Check sheet for the modelled part. Datum: model origin and axes. Units: mm. A direction names the side the tool comes from. Round coordinates to 2 decimals unless told otherwise and drop trailing zeros. Write each loop counter-clockwise with the first axis right and the second up, starting at its lowest first coordinate (ties: lowest second). Pieces come first, ordered by that corner, then holes. Notation, with made-up numbers: (41.25, -9.75) -> (52.25, -9.75) arc R20 ccw to (52.25, 4.25) -> close; hole circle Ø5 at (37, 17.5). An arc over 180 degrees is marked (long way). One line per item, written item: value.
from build123d import *

# Parameters (mm, degrees)
BOSS_EXTRUDE1_DEPTH = 5
SKETCH2_R           = 7.075
SKETCH2_R_2         = 2
CUT_EXTRUDE1_DEPTH  = 5
FILLET1_R           = 10
FILLET2_R           = 10


with BuildPart() as part:
    # Sketch1 → Boss-Extrude1 (new body)
    with BuildSketch(Plane(origin=(0, 0, 0), x_dir=(1, 0, 0), z_dir=(0, 1, 0))):
        Polygon((-40.926174497, 16.946308725), (-88.926174497, 16.946308725), (-88.926174497, -33.053691275), (-40.926174497, -33.053691275), (-40.926174497, -8.053691275), (-30.926174497, -8.053691275), (-13.571066073, -8.053691275), (21.073825503, -8.053691275), (21.073825503, 46.946308725), (-30.926174497, 46.946308725), (-40.926174497, 46.946308725), align=None)
    extrude(amount=BOSS_EXTRUDE1_DEPTH)

    # Sketch2 → Cut-Extrude1 (cut)
    with BuildSketch(Plane(origin=(0, 5, 0), x_dir=(1, 0, 0), z_dir=(0, 1, 0))):
        with Locations(Location((-64.926174497, -9.053691275, 0), (0, 0, 270))):
            Circle(SKETCH2_R)
        with Locations(Location((-72.926174497, -1.053691275, 0), (0, 0, 270))):
            Circle(SKETCH2_R_2)
        with Locations(Location((-56.926174497, -1.053691275, 0), (0, 0, 270))):
            Circle(SKETCH2_R_2)
        with Locations(Location((-56.926174497, -17.053691275, 0), (0, 0, 270))):
            Circle(SKETCH2_R_2)
        with Locations(Location((-72.926174497, -17.053691275, 0), (0, 0, 270))):
            Circle(SKETCH2_R_2)
        with Locations(Location((-2.926174497, 23.643183553, 0), (0, 0, 270))):
            Circle(SKETCH2_R)
        with Locations(Location((5.073825503, 31.643183553, 0), (0, 0, 270))):
            Circle(SKETCH2_R_2)
        with Locations(Location((-10.926174497, 15.643183553, 0), (0, 0, 270))):
            Circle(SKETCH2_R_2)
        with Locations(Location((-10.926174497, 31.643183553, 0), (0, 0, 270))):
            Circle(SKETCH2_R_2)
        with Locations(Location((5.073825503, 15.643183553, 0), (0, 0, 270))):
            Circle(SKETCH2_R_2)
    extrude(amount=-CUT_EXTRUDE1_DEPTH, mode=Mode.SUBTRACT)

    # Fillet1
    fillet1_edges = [part.edges().sort_by_distance(p)[0] for p in [
        (-88.926174497, 2.5, -16.946308725),
    ]]
    fillet(fillet1_edges, radius=FILLET1_R)

    # Fillet2
    fillet2_edges = [part.edges().sort_by_distance(p)[0] for p in [
        (21.073825503, 2.5, -46.946308725),
        (21.073825503, 2.5, 8.053691275),
        (-40.926174497, 2.5, 8.053691275),
        (-40.926174497, 2.5, 33.053691275),
        (-88.926174497, 2.5, 33.053691275),
        (-40.926174497, 2.5, -16.946308725),
        (-40.926174497, 2.5, -46.946308725),
    ]]
    fillet(fillet2_edges, radius=FILLET2_R)


solid = part.part
Item 1: Sectioned sample at B-B (z = -22.5). Enter the section's corners in (x, y).
Result set:
outline: (-41.97, 0) -> (-9.91, 0) -> (-9.91, 5) -> (-41.97, 5) -> close; (4.06, 0) -> (21.07, 0) -> (21.07, 5) -> (4.06, 5) -> close
Item 2: Sectioned sample at D-D (x = -23.5). Enter the section's corners in (y, z).
Result set:
outline: (0, -46.95) -> (5, -46.95) -> (5, 8.05) -> (0, 8.05) -> close
Item 3: Release check for a two-part mould opening along Z. For faces 1 (the flat face through (-40.926, 2, 21)), 2 (the cylindrical face through (-71.2, 2.54, 12.32)), 3 (the cylindrical face through (-43.93, 2.54, 30.2)) record: pulls with the +Z half, pulls with the -Z half, needs draft (parallel to the pull), parting line crosses it, or undercut.
Result set:
face 1: needs draft
face 2: undercut
face 3: pulls with the +Z half
Item 4: Material ranges on line 1 along X through (y, z) = (3, 18); line 2 along X through (y, z) = (0.3, -14); line 3 along Z through (x, y) = (-15.5, 1.4), recorded low to high.
Result set:
line 1: -88.93 to -74.69, -71.16 to -58.69, -55.16 to -40.93
line 2: -86.01 to -12.07, -9.79 to 3.93, 6.21 to 21.07
line 3: -46.95 to 8.05
Item 5: Sectioned sample at A-A (x = 1). Enter the section's corners in (y, z).
Result set:
outline: (0, -46.95) -> (5, -46.95) -> (5, -29.53) -> (0, -29.53) -> close; (0, -17.76) -> (5, -17.76) -> (5, 8.05) -> (0, 8.05) -> close
Item 6: Tool access check on faces 4 (the flat face through (-40.926, 2, -32)), 5 (the flat face through (-88.926, 2, 8)), 6 (the flat face through (-10, 2, 8.054)). Record the directions out of +Z, -Z, +X, -X, +Y, -Y that give a thin tool (end or side, any length) a straight path to the whole face; none if there is none.
Result set:
face 4: -Z, -X, +Y, -Y
face 5: +Z, -Z, -X, +Y, -Y
face 6: +Z, +X, +Y, -Y
Item 7: Depth check by flat-ended pin: pin 1 (3 mm diameter, centred on x = -10.93, z = -31.64, fed in from +Y); pin 2 (1.5 mm diameter, centred on y = 3.5, z = 21.5, fed in from +X); pin 3 (1.5 mm diameter, centred on y = 3.5, z = -31.5, fed in from -X); pin 4 (3 mm diameter, centred on x = -52.5, y = 3.5, fed in from -Z). Enter the tip coordinate at first touch or a pass-through.
Result set:
pin 1: through
pin 2: x = -40.93
pin 3: x = -40.93
pin 4: z = -16.95
Item 8: Sectioned sample at C-C (y = 2.65). State how many separate pieces and enclosed holes the cut face has, then the cut area to 3 significant figures.
Result set:
separate pieces: 1
enclosed holes: 10
area: 5,310 mm^2
